```python
from build123d import *

# Parameters (mm, degrees)
SKETCH_1_W          = 250
SKETCH_1_H          = 30
SKETCH_1_R          = 1.5
EXTRUDE_1_DEPTH     = 4
SKETCH_2_R          = 3
CUT_EXTRUDE_1_DEPTH = 126.96031121
SKETCH_3_W          = 250
SKETCH_3_H          = 70
SKETCH_3_R          = 1.5
SKETCH_3_R_2        = 2.1
EXTRUDE_2_DEPTH     = 4
CUT_EXTRUDE_2_DEPTH = 152.215078613
FILLET_1_R          = 5
SKETCH_5_R          = 3
CUT_EXTRUDE_3_DEPTH = 152.215078613
SKETCH_8_W          = 20
SKETCH_8_H          = 50
EXTRUDE_4_DEPTH     = 4
SKETCH_9_R          = 1
CUT_EXTRUDE_4_DEPTH = 10
SKETCH_10_W         = 35
SKETCH_10_H         = 30
CUT_EXTRUDE_5_DEPTH = 10
SKETCH_11_W         = 70
SKETCH_11_H         = 4.604086331
EXTRUDE_5_DEPTH     = 4
FILLET_4_R          = 10
CUT_EXTRUDE_6_DEPTH = 10
SKETCH_14_W         = 11.507162467
SKETCH_14_H         = 5
EXTRUDE_6_DEPTH     = 4
SKETCH_15_W         = 3
SKETCH_15_H         = 55
SKETCH_15_W_2       = 15
SKETCH_15_H_2       = 50
CUT_EXTRUDE_7_DEPTH = 10
FILLET_6_R          = 3
SKETCH_16_R         = 1.6
CUT_EXTRUDE_8_DEPTH = 10
CHAMFER_2_SIZE      = 1


with BuildPart() as part:
    # 草图1 → 凸台-拉伸1 (new body)
    with BuildSketch(Plane.XY):
        Rectangle(SKETCH_1_W, SKETCH_1_H)
        with Locations((-115, -10)):
            Circle(SKETCH_1_R, mode=Mode.SUBTRACT)
        with Locations((-115, 10)):
            Circle(SKETCH_1_R, mode=Mode.SUBTRACT)
        with Locations(Location((115, 10, 0), (0, 0, 180))):
            Circle(SKETCH_1_R, mode=Mode.SUBTRACT)
        with Locations(Location((115, -10, 0), (0, 0, 180))):
            Circle(SKETCH_1_R, mode=Mode.SUBTRACT)
    extrude(amount=EXTRUDE_1_DEPTH)

    # 草图2 → 切除-拉伸1 (cut, through all)
    with BuildSketch(Plane.XY.offset(4)):
        with Locations((-23, 2.5)):
            Circle(SKETCH_2_R)
        with Locations((23, 2.5)):
            Circle(SKETCH_2_R)
        with Locations((23, 15.5)):
            Circle(SKETCH_2_R)
        with Locations((-23, 15.5)):
            Circle(SKETCH_2_R)
    extrude(amount=-CUT_EXTRUDE_1_DEPTH, mode=Mode.SUBTRACT)

    # 草图3 → 凸台-拉伸2 (add)
    with BuildSketch(Plane.XY.offset(4)):
        with Locations((0, 50)):
            Rectangle(SKETCH_3_W, SKETCH_3_H)
        with Locations((-115, 30)):
            Circle(SKETCH_3_R, mode=Mode.SUBTRACT)
        with Locations((-115, 50)):
            Circle(SKETCH_3_R, mode=Mode.SUBTRACT)
        with Locations((-115, 70)):
            Circle(SKETCH_3_R, mode=Mode.SUBTRACT)
        with Locations((115, 30)):
            Circle(SKETCH_3_R, mode=Mode.SUBTRACT)
        with Locations((115, 50)):
            Circle(SKETCH_3_R, mode=Mode.SUBTRACT)
        with Locations((115, 70)):
            Circle(SKETCH_3_R, mode=Mode.SUBTRACT)
        with Locations((-35, 77.5)):
            Circle(SKETCH_3_R_2, mode=Mode.SUBTRACT)
        with Locations((35, 77.5)):
            Circle(SKETCH_3_R_2, mode=Mode.SUBTRACT)
    extrude(amount=-EXTRUDE_2_DEPTH)

    # 草图4 → 切除-拉伸2 (cut, through all)
    with BuildSketch(Plane.XY.offset(4)):
        with BuildLine():
            Line((-97, 70), (-48, 70))
            ThreePointArc((-48, 70), (-45.878679656, 69.121320344), (-45, 67))
            Line((-45, 67), (-45, 3))
            ThreePointArc((-45, 3), (-45.878679656, 0.878679656), (-48, 0))
            Line((-48, 0), (-97, 0))
            ThreePointArc((-97, 0), (-99.121320344, 0.878679656), (-100, 3))
            Line((-100, 3), (-100, 67))
            ThreePointArc((-100, 67), (-99.121320344, 69.121320344), (-97, 70))
        make_face()
        with BuildLine():
            Line((97, 0), (48, 0))
            ThreePointArc((48, 0), (45.878679656, 0.878679656), (45, 3))
            Line((45, 3), (45, 67))
            ThreePointArc((45, 67), (45.878679656, 69.121320344), (48, 70))
            Line((48, 70), (97, 70))
            ThreePointArc((97, 70), (99.121320344, 69.121320344), (100, 67))
            Line((100, 67), (100, 3))
            ThreePointArc((100, 3), (99.121320344, 0.878679656), (97, 0))
        make_face()
    extrude(amount=-CUT_EXTRUDE_2_DEPTH, mode=Mode.SUBTRACT)

    # 圆角1
    fillet_1_edges = [part.edges().sort_by_distance(p)[0] for p in [
        (125, 85, 2),
        (-125, 85, 2),
        (125, -15, 2),
        (-125, -15, 2),
    ]]
    fillet(fillet_1_edges, radius=FILLET_1_R)

    # 草图5 → 切除-拉伸3 (cut, through all)
    with BuildSketch(Plane.XY.offset(4)):
        with Locations((-23, 15.5)):
            Circle(SKETCH_5_R)
        with Locations((23, 15.5)):
            Circle(SKETCH_5_R)
    extrude(amount=-CUT_EXTRUDE_3_DEPTH, mode=Mode.SUBTRACT)

    # 草图8 → 凸台-拉伸4 (add)
    with BuildSketch(Plane.XY.offset(4)):
        with Locations((-55, 45)):
            Rectangle(SKETCH_8_W, SKETCH_8_H)
    extrude(amount=-EXTRUDE_4_DEPTH)

    # 草图9 → 切除-拉伸4 (cut)
    with BuildSketch(Plane.XY.offset(4)):
        with Locations((-47, 22)):
            Circle(SKETCH_9_R)
        with Locations((-29, 22)):
            Circle(SKETCH_9_R)
        with Locations((-47, 67.2)):
            Circle(SKETCH_9_R)
        with Locations((-29, 67.2)):
            Circle(SKETCH_9_R)
    extrude(amount=-CUT_EXTRUDE_4_DEPTH, mode=Mode.SUBTRACT)

    # 草图10 → 切除-拉伸5 (cut)
    with BuildSketch(Plane.XY.offset(4)):
        with Locations((-17.5, 0)):
            Rectangle(SKETCH_10_W, SKETCH_10_H)
        with Locations((17.5, 0)):
            Rectangle(SKETCH_10_W, SKETCH_10_H)
    extrude(amount=-CUT_EXTRUDE_5_DEPTH, mode=Mode.SUBTRACT)

    # 草图11 → 凸台-拉伸5 (add)
    with BuildSketch(Plane.XY.offset(4)):
        with Locations((0, 17.302043166)):
            Rectangle(SKETCH_11_W, SKETCH_11_H)
    extrude(amount=-EXTRUDE_5_DEPTH)

    # 圆角4
    fillet_4_edges = [part.edges().sort_by_distance(p)[0] for p in [
        (-35, -15, 2),
        (35, -15, 2),
        (35, 15, 2),
        (-35, 15, 2),
    ]]
    fillet(fillet_4_edges, radius=FILLET_4_R)

    # 草图12 → 切除-拉伸6 (cut)
    with BuildSketch(Plane.XY.offset(4)):
        Polygon((-159.482057717, 67), (-159.482057717, -21.443198138), (-25, -21.443198138), (-25, 15), (-56.507162467, 15), (-56.507162467, 102.331531395), (-144.590660761, 102.331531395), (-144.590660761, 67), align=None)
        Polygon((45, 102.331531395), (45, 15), (25, 15), (25, -21.443198138), (159.482057717, -21.443198138), (159.482057717, 67), (144.590660761, 67), (144.590660761, 102.331531395), align=None)
    extrude(amount=-CUT_EXTRUDE_6_DEPTH, mode=Mode.SUBTRACT)

    # 草图14 → 凸台-拉伸6 (add)
    with BuildSketch(Plane.XY.offset(4)):
        with Locations((-50.753581234, 17.5)):
            Rectangle(SKETCH_14_W, SKETCH_14_H)
    extrude(amount=-EXTRUDE_6_DEPTH)

    # 草图15 → 切除-拉伸7 (cut)
    with BuildSketch(Plane.XY.offset(4)):
        Polygon((-56.507162467, 70), (-53.507162467, 70), (-46.507162467, 70), (-46.507162467, 85), (-56.507162467, 85), align=None)
        with Locations((-55.007162467, 42.5)):
            Rectangle(SKETCH_15_W, SKETCH_15_H)
        with Locations((37.5, 40)):
            Rectangle(SKETCH_15_W_2, SKETCH_15_H_2)
    extrude(amount=-CUT_EXTRUDE_7_DEPTH, mode=Mode.SUBTRACT)

    # 圆角6
    fillet_6_edges = [part.edges().sort_by_distance(p)[0] for p in [
        (45, 85, 2),
        (30, 15, 2),
        (-46.507162467, 70, 2),
        (-46.507162467, 85, 2),
        (-53.507162467, 70, 2),
        (-53.507162467, 15, 2),
        (30, 65, 2),
        (45, 65, 2),
    ]]
    fillet(fillet_6_edges, radius=FILLET_6_R)

    # 草图16 → 切除-拉伸8 (cut)
    with BuildSketch(Plane.XY.offset(4)):
        with Locations((-7.5, 42.2)):
            Circle(SKETCH_16_R)
        with Locations((7.5, 42.2)):
            Circle(SKETCH_16_R)
        with Locations((-7.5, 22.2)):
            Circle(SKETCH_16_R)
        with Locations((7.5, 22.2)):
            Circle(SKETCH_16_R)
    extrude(amount=-CUT_EXTRUDE_8_DEPTH, mode=Mode.SUBTRACT)

    # 倒角2
    chamfer_2_edges = [part.edges().sort_by_distance(p)[0] for p in [
        (-9.1, 42.2, 0),
    ]]
    chamfer(chamfer_2_edges, length=CHAMFER_2_SIZE)


solid = part.part
```
Work out the finished part from the listing and answer in its coordinate system (mm). A direction names the side the tool comes from. Give positions to 0.01 mm unless a question says otherwise; leave off trailing zeros. Loops run counter-clockwise (first coordinate to the right, second up) from the corner with the lowest first, then second, coordinate; pieces in that order, holes last. Notation, with made-up numbers: (68, 55) - (109, 55) arc R36 ccw to (109, 94) - close; hole circle Ø8 at (3, -30.5). An arc over 180 degrees is marked (long way). Use CSV: the item, a comma, the result in double quotes. Start each with the question number.
(1) Find section C-C, the plane x = -35. Determine the outline of the cut face in (y, z), plus the area to 3 significant figures.
(2) A tool of negligible diameter and unlimited length cuts with its end or side. For faces 1 (the face through (-46.507, 77, 2)), 2 (the face through (37, 65, 2)), 3 (the face through (-46, 22, 2)), from which of +Z, -Z, +X, -X, +Y, -Y can it reach the whole face along a straight path? Write none if from no direction.
(3) Find section A-A, the plane x = -7.5. Determine the outline of the cut face in (y, z), plus the area to 3 significant figures.
(4) Find the intervals of material crossed by L1, parallel to Y at x = 7.5, z = 2.55; L2, parallel to Y at x = -29, z = 2.1; L3, parallel to Y at x = 35, z = 2.7, in increasing order.
(5) Determine the mould class of faces 4 (the face through (44.14, 65.9, 1.97)), 5 (the face through (-5, 50, 0)), 6 (the face through (7.15, 20.64, 2.03)) for opening direction Y: released by +Y, released by -Y, zero draft, split by the parting line, or undercut.
(6) Each of these flat-tipped pins is pushed along its axis until it touches: pin 1 (5 mm diameter, centred on x = 7.5, y = 42.2, fed in from +Z); pin 2 (1.2 mm diameter, centred on x = -47, y = 22, fed in from -Z); pin 3 (2 mm diameter, centred on x = 39.5, z = 1.5, fed in from -Y); pin 4 (1.2 mm diameter, centred on y = 44, z = 2.5, fed in from +X). Where does it stop, or does it pass through?
(7) Find section B-B, the plane y = 77.5. Determine the outline of the cut face in (x, z), plus the area to 3 significant figures.
(8) Find section D-D, the plane z = 3. Count the separate pieces of the cut face and the enclosed holes in it, plus the area to 3 significant figures.
Results found:
1,outline,"(15, 0) - (75.4, 0) - (75.4, 4) - (15, 4) - close; (79.6, 0) - (85, 0) - (85, 4) - (79.6, 4) - close"
1,area,"263 mm^2"
2,face 1,"+Z, -Z, -X, +Y"
2,face 2,"+Z, -Z, +X, -Y"
2,face 3,"+Z, -Z"
3,outline,"(15, 0) - (20.6, 0) - (20.6, 4) - (15, 4) - close; (23.8, 0) - (39.6, 0) - (40.6, 1) - (40.6, 4) - (23.8, 4) - close; (43.8, 1) - (44.8, 0) - (85, 0) - (85, 4) - (43.8, 4) - close"
3,area,"253 mm^2"
4,L1,"15 to 20.6, 23.8 to 40.6, 43.8 to 85"
4,L2,"15 to 21, 23 to 66.2, 68.2 to 85"
4,L3,"65 to 75.4, 79.6 to 85"
5,face 4,"released by -Y"
5,face 5,"zero draft"
5,face 6,"undercut"
6,pin 1,"z = 4"
6,pin 2,"through"
6,pin 3,"y = 65"
6,pin 4,"x = 30"
7,outline,"(-46.51, 0) - (-37.1, 0) - (-37.1, 4) - (-46.51, 4) - close; (-32.9, 0) - (32.9, 0) - (32.9, 4) - (-32.9, 4) - close; (37.1, 0) - (45, 0) - (45, 4) - (37.1, 4) - close"
7,area,"332 mm^2"
8,separate pieces,"1"
8,enclosed holes,"10"
8,area,"5,960 mm^2"
